Geometry check sheet. Reference: the model listing, model coordinates, mm. Face numbers are marked on the shaded views. Round coordinates to 2 decimals unless told otherwise and drop trailing zeros. Loops run counter-clockwise (first coordinate to the right, second up) from the corner with the lowest first, then second, coordinate; pieces in that order, holes last. Notation, with made-up numbers: (88.25, -24.75) -> (93.25, -24.75) arc R10 cw to (93.25, -9.75) -> close; hole circle Ø5 at (-8, 45.25). An arc over 180 degrees is marked (long way). Use one line per item in the form item = value.
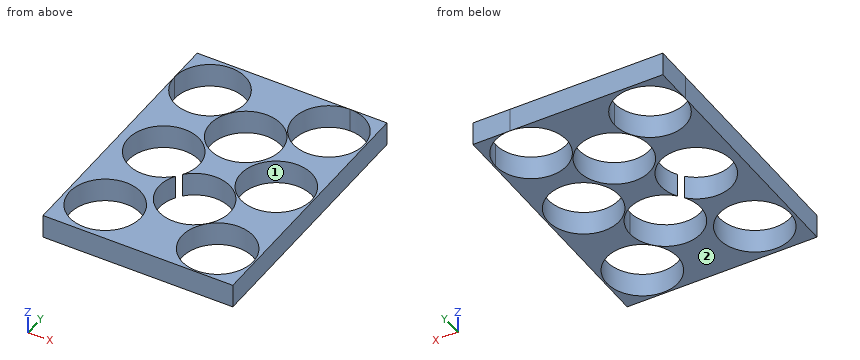
Autodesk Inventor part; units mm, degrees
ref_plane "YZ Plane" through (0, 0, 0) normal (1, 0, 0) x (0, 1, 0)
ref_plane "XZ Plane" through (0, 0, 0) normal (0, 1, 0) x (-1, 0, 0)
ref_plane "XY Plane" through (0, 0, 0) normal (0, 0, 1) x (1, 0, 0)
sketch "Sketch1" plane through (0, 0, 0) normal (0, 0, 1) x (1, 0, 0)
  line L0 (0, 0) -> (0, 279.4)
  line L1 (0, 279.4) -> (203.2, 279.4)
  line L2 (203.2, 279.4) -> (203.2, 0)
  line L3 (203.2, 0) -> (0, 0)
  circle A0 centre (101.6, 195.2625) radius 38.1
  circle A1 centre (163.5125, 39.6875) radius 38.1
  circle A2 centre (41.275, 42.8625) radius 38.1
  circle A3 centre (107.95, 92.075) radius 38.1
  circle A4 centre (163.5125, 146.05) radius 38.1
  circle A5 centre (47.625, 138.1125) radius 38.1
  circle A6 centre (38.1, 238.125) radius 38.1
  circle A7 centre (163.5125, 241.3) radius 38.1
  dimension "d0" = 203.2
  dimension "d1" = 279.4
  dimension "d2" = 76.2
  dimension "d3" = 76.2
  dimension "d4" = 76.2
  dimension "d5" = 76.2
  dimension "d6" = 76.2
  dimension "d7" = 76.2
  dimension "d8" = 76.2
  dimension "d9" = 76.2
extrude "Extrusion1" add sketch "Sketch1" along normal blind 25.4
properties part number "5.1 Q6"
1. Section check A-A (x = 185). Record the boundary of the cut face in (y, z), then the cut area to 3 significant figures.
Return value:
outline = (0, 0) -> (8.22, 0) -> (8.22, 25.4) -> (0, 25.4) -> close; (71.15, 0) -> (114.59, 0) -> (114.59, 25.4) -> (71.15, 25.4) -> close; (177.51, 0) -> (209.84, 0) -> (209.84, 25.4) -> (177.51, 25.4) -> close; (272.76, 0) -> (279.4, 0) -> (279.4, 25.4) -> (272.76, 25.4) -> close
area = 2,300 mm2
2. Mould release check, pull along X, two halves, no side actions. Record for the marked faces 1 and 2: released by +X, released by -X, zero draft, split by the parting line, or undercut.
Return value:
face_1 = undercut
face_2 = zero draft
3. Section check C-C (y = 146.05). Record the boundary of the cut face in (x, z).
Return value:
outline = (0, 0) -> (10.36, 0) -> (10.36, 25.4) -> (0, 25.4) -> close; (84.89, 0) -> (125.41, 0) -> (125.41, 25.4) -> (84.89, 25.4) -> close; (201.61, 0) -> (203.2, 0) -> (203.2, 25.4) -> (201.61, 25.4) -> close
4. Material ranges on line 1 along X through (y, z) = (233.5, 15.25); line 2 along Y through (x, z) = (128.5, 20.75); line 3 along Y through (x, z) = (69.5, 14), recorded low to high.
Return value:
line_1 = 0 to 0.28, 75.92 to 126.22, 200.81 to 203.2
line_2 = 0 to 24.66, 54.71 to 59.99, 124.16 to 131.03, 161.07 to 168.28, 222.24 to 226.28, 256.32 to 279.4
line_3 = 0 to 17.27, 68.45 to 106.92, 169.31 to 174.74, 215.79 to 216.55, 259.7 to 279.4
5. Section check B-B (y = 214). Record the boundary of the cut face in (x, z).
Return value:
outline = (0, 0) -> (8.61, 0) -> (8.61, 25.4) -> (0, 25.4) -> close; (67.59, 0) -> (68.43, 0) -> (68.43, 25.4) -> (67.59, 25.4) -> close; (134.77, 0) -> (136.94, 0) -> (136.94, 25.4) -> (134.77, 25.4) -> close; (190.09, 0) -> (203.2, 0) -> (203.2, 25.4) -> (190.09, 25.4) -> close
